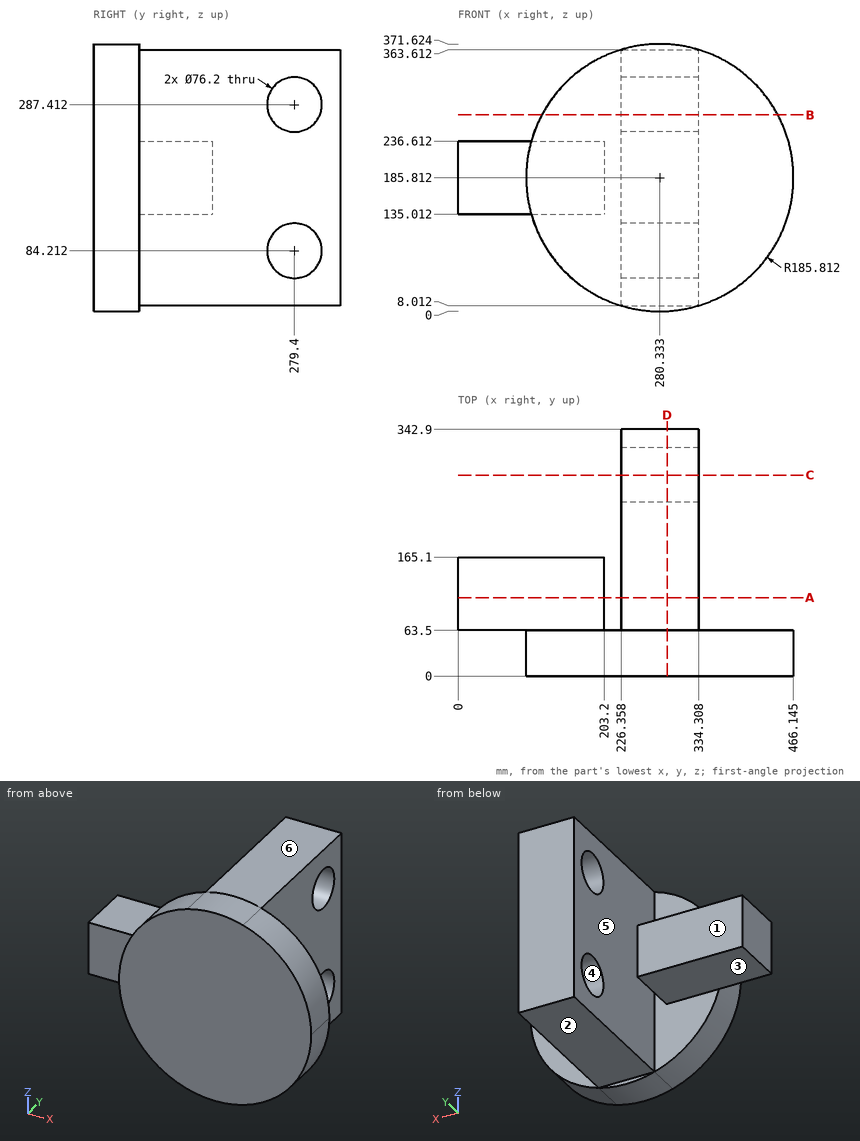
Verification items for this drawing (mm, ordinates from the low corner). A direction names the side the tool comes from. Round coordinates to 2 decimals unless told otherwise and drop trailing zeros. Order: outer loops, then holes, each group sorted by start corner. A loop starts at its lowest first (then second) coordinate and runs counter-clockwise, first axis right, second up.
1) Depth check by flat-ended pin: pin 1 (8 mm diameter, centred on y = 44.5, z = 76, fed in from -X); pin 2 (8 mm diameter, centred on y = 37.5, z = 156, fed in from +X); pin 3 (5 mm diameter, centred on y = 199.5, z = 237.5, fed in from -X). Enter the tip coordinate at first touch or a pass-through.
Geometry says:
pin 1: stops at x = 127.59
pin 2: stops at x = 464.34
pin 3: stops at x = 226.36
2) Tool access check on the marked faces 1, 2 and 3. Record the directions out of +Z, -Z, +X, -X, +Y, -Y that give a thin tool (end or side, any length) a straight path to the whole face; none if there is none.
Geometry says:
face 1: +Z, -Z, -X, +Y
face 2: -Z, +X, -X, +Y
face 3: -Z, -X, +Y
3) Material ranges on line 1 (Z direction, x = 286, y = 279); line 2 (Y direction, x = 200, z = 275.5); line 3 (Z direction, x = 315.5, y = 146.5), recorded low to high.
Geometry says:
line 1: z = 8.01 to 46.11, 122.31 to 249.31, 325.51 to 363.61
line 2: y = 0 to 63.5
line 3: z = 8.01 to 363.61
4) Draft check along Z on the marked faces 4, 5 and 6. Enter one of: +Z half, -Z half, draft (parallel to the pull), parting line (faces both ways), or undercut.
Geometry says:
face 4: undercut
face 5: draft
face 6: +Z half
5) Cross-section at B-B, the plane z = 273. Record the cut outline in (x, y).
Geometry says:
outline: (116.25, 0) - (444.42, 0) - (444.42, 63.5) - (334.31, 63.5) - (334.31, 244.13) - (226.36, 244.13) - (226.36, 63.5) - (116.25, 63.5) - close; (226.36, 314.67) - (334.31, 314.67) - (334.31, 342.9) - (226.36, 342.9) - close
6) Cross-section at A-A, the plane y = 109. Record the cut outline in (x, z).
Geometry says:
outline: (0, 135.01) - (203.2, 135.01) - (203.2, 236.61) - (0, 236.61) - close; (226.36, 8.01) - (334.31, 8.01) - (334.31, 363.61) - (226.36, 363.61) - close
7) Cross-section at C-C, the plane y = 279.4. Record the cut outline in (x, z), plus the area to 3 significant figures.
Geometry says:
outline: (226.36, 8.01) - (334.31, 8.01) - (334.31, 46.11) - (226.36, 46.11) - close; (226.36, 122.31) - (334.31, 122.31) - (334.31, 249.31) - (226.36, 249.31) - close; (226.36, 325.51) - (334.31, 325.51) - (334.31, 363.61) - (226.36, 363.61) - close
area: 21,900 mm2
8) Cross-section at D-D, the plane x = 290.5. Record the cut outline in (y, z), plus the area to 3 significant figures.
Geometry says:
outline: (0, 0.28) - (63.5, 0.28) - (63.5, 8.01) - (342.9, 8.01) - (342.9, 363.61) - (63.5, 363.61) - (63.5, 371.35) - (0, 371.35) - close; hole circle Ø76.2 at (279.4, 84.21); hole circle Ø76.2 at (279.4, 287.41)
area: 114,000 mm2
